For this review, take the finished solid that the model builds, in its own axes (mm). Coordinates: 2 decimals unless noted, no trailing zeros. Order: outer loops, then holes, each group sorted by start corner. A loop starts at its lowest first (then second) coordinate and runs counter-clockwise, first axis right, second up. Notation, with made-up numbers: M 18,-38 L 72,-38 A18 ccw 72,-8 Z; hole C 20,70 d11. An arc over 180 degrees is marked long. Use one line per item in the form item = value. Start each with the question number.
```python
from build123d import *

# Parameters (mm, degrees)
F0_R     = 10
F0_R_2   = 9.5
F1_DEPTH = 3.3
F0_R_3   = 5
F2_DEPTH = 3
F3_DEPTH = 25


with BuildPart() as f1:
    # F0 (on Front) → F1 (new body)
    with BuildSketch(Plane.XZ):
        Circle(F0_R)
        Circle(F0_R_2, mode=Mode.SUBTRACT)
    extrude(amount=F1_DEPTH)

    # F0 (on Front) → F2 (join)
    with BuildSketch(Plane.XZ):
        Circle(F0_R_2)
        Circle(F0_R_3, mode=Mode.SUBTRACT)
        Circle(F0_R_3)
    extrude(amount=F2_DEPTH)

    # F0 (on Front) → F3 (cut)
    with BuildSketch(Plane.XZ):
        Circle(F0_R_3)
    extrude(amount=F3_DEPTH, mode=Mode.SUBTRACT)


solid = f1.part
```
1. To check wall thickness, follow line 1 (Z direction, x = 0, y = -2); line 2 (Z direction, x = 0, y = -3.2); line 3 (Y direction, x = -7, z = 0.75). State the ranges of each line that lie inside material, in increasing order.
2. Consider section A-A, the plane z = 0. Write out the cut boundary in (x, y).
3. Consider section C-C, the plane y = -1. Write out the cut boundary in (x, z), plus the area to 3 significant figures.
4. Consider section D-D, the plane z = 6. Write out the cut boundary in (x, y), plus the area to 3 significant figures.
5. For pin 1 Ø1.5 at (y, z) = (-1, -4) entering from -X; pin 2 Ø8 at (x, z) = (0, 0) entering from +Y; pin 3 Ø5.5 at (x, z) = (4, 1.5) entering from -Y; pin 4 Ø1 at (x, y) = (-1, -1) entering from -Z, all flat-tipped, find the tip position at first contact; note any pin that passes through.
6. The part is to be moulded in two halves that separate along Z. For faces 1 (the flat face through (2, 0, 5)), 2 (the flat face through (4, -3, -4)), 3 (the cylindrical face through (-1.08, -1.48, -4.88)), 4 (the cylindrical face through (-2.17, -1.63, -9.76)), say which applies: pulls with the +Z half, pulls with the -Z half, needs draft (parallel to the pull), parting line crosses it, or undercut.
7. Consider section B-B, the plane x = 0. Write out the cut boundary in (y, z), plus the area to 3 significant figures.
Answers follow:
q1.line_1 = -10 to -5, 5 to 10
q1.line_2 = -10 to -9.5, 9.5 to 10
q1.line_3 = -3 to 0
q2.outline = M -10,-3.3 L -9.5,-3.3 L -9.5,-3 L -5,-3 L -5,0 L -10,0 Z; M 5,-3 L 9.5,-3 L 9.5,-3.3 L 10,-3.3 L 10,0 L 5,0 Z
q3.outline = C 0,0 d20; hole C 0,0 d10
q3.area = 236 mm²
q4.outline = M -8,-3.3 L -7.37,-3.3 L -7.37,-3 L 7.37,-3 L 7.37,-3.3 L 8,-3.3 L 8,0 L -8,0 Z
q4.area = 48.4 mm²
q5.pin_1 = -9.46
q5.pin_2 = through
q5.pin_3 = -3
q5.pin_4 = -9.99
q6.face_1 = needs draft
q6.face_2 = undercut
q6.face_3 = undercut
q6.face_4 = parting line crosses it
q7.outline = M -3.3,-10 L 0,-10 L 0,-5 L -3,-5 L -3,-9.5 L -3.3,-9.5 Z; M -3.3,9.5 L -3,9.5 L -3,5 L 0,5 L 0,10 L -3.3,10 Z
q7.area = 30.3 mm²
